Geometry: see drawing. Coordinates: mm, zero at the bounding-box minimum. A direction names the side the tool comes from. Give positions to 0.01 mm unless a question says otherwise; leave off trailing zeros. Write each loop counter-clockwise with the first axis right and the second up, starting at its lowest first coordinate (ties: lowest second). Pieces come first, ordered by that corner, then holes.
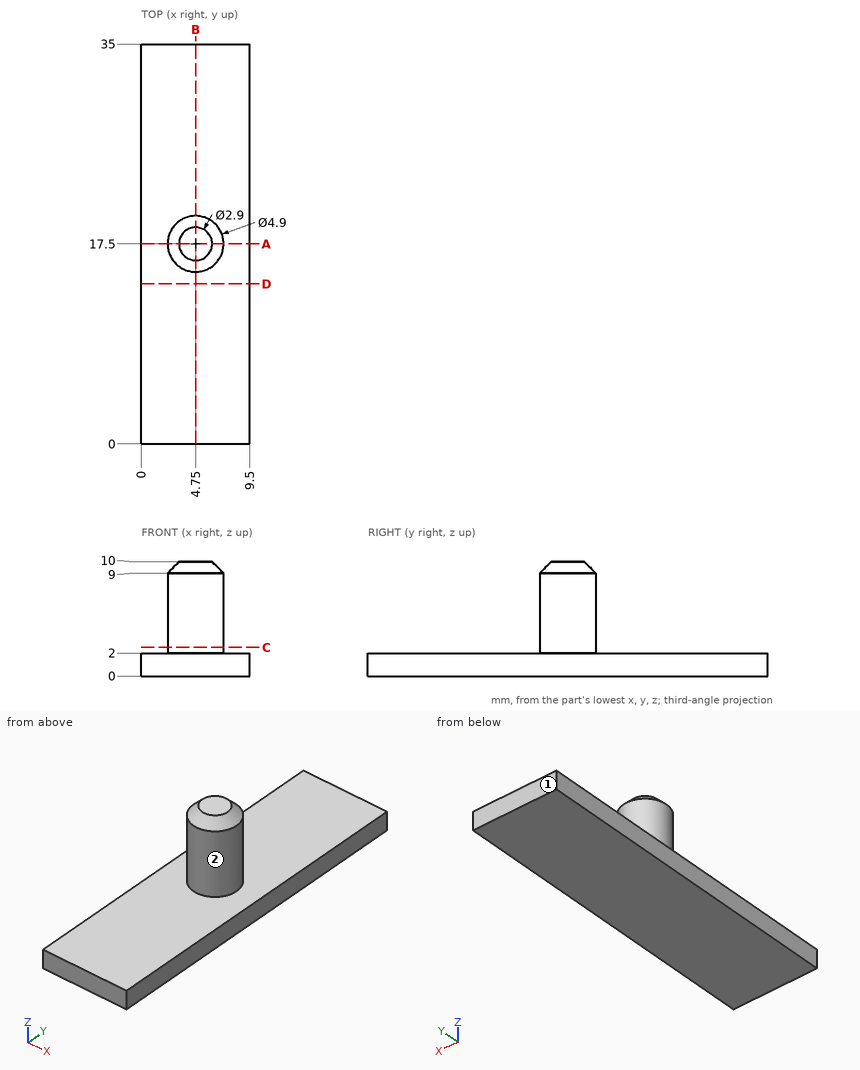
1. Line query: probe 1 along Z at (x, y) = (7.75, 24); probe 2 along Y at (x, z) = (4.75, 4); probe 3 along Y at (x, z) = (5.5, 8.25). Output: solid intervals per line, ascending.
2. Access query for the marked faces 1 and 2. Directions: +Z, -Z, +X, -X, +Y, -Y. A direction counts if a zero-diameter tool reaches every point of the face in a straight line with its end or side. Return the directions, or none.
3. Pin query (flat end, axial travel): P1, Ø5, axis at x = 3.5, z = 6, coming from the -Y side; P2, Ø5, axis at x = 1.5, y = 31.5, coming from the +Z side. Return the tip coordinate at first contact, or that it passes through.
4. Section query A-A (y = 17.5). Return loops of the section in (x, z).
5. Section query B-B (x = 4.75). Return loops of the section in (y, z).
6. Section query D-D (y = 14). Return loops of the section in (x, z), plus the area to 3 significant figures.
7. Section query C-C (z = 2.5). Return loops of the section in (x, y), plus the area to 3 significant figures.
The answers:
1. probe 1: z = 0 to 2
1. probe 2: y = 15.05 to 19.95
1. probe 3: y = 15.17 to 19.83
2. face 1: +Z, -Z, +X, -X, +Y
2. face 2: +Z
3. P1: stops at y = 15.05
3. P2: stops at z = 2
4. outline: (0, 0) - (9.5, 0) - (9.5, 2) - (7.2, 2) - (7.2, 9) - (6.2, 10) - (3.3, 10) - (2.3, 9) - (2.3, 2) - (0, 2) - close
5. outline: (0, 0) - (35, 0) - (35, 2) - (19.95, 2) - (19.95, 9) - (18.95, 10) - (16.05, 10) - (15.05, 9) - (15.05, 2) - (0, 2) - close
6. outline: (0, 0) - (9.5, 0) - (9.5, 2) - (0, 2) - close
6. area: 19.0 mm2
7. outline: circle Ø4.9 at (4.75, 17.5)
7. area: 18.9 mm2
